```python
from build123d import *

# Parameters (mm, degrees)
F0_R     = 5
F1_DEPTH = 5
F2_R     = 1
F3_DEPTH = 1


with BuildPart() as f1:
    # F0 (on Front) → F1 (new body)
    with BuildSketch(Plane.XZ):
        with BuildLine():
            ThreePointArc((9.943923, -1.057539), (9.985971, -0.529512), (10, 0))
            ThreePointArc((10, 0), (9.985971, 0.529512), (9.943923, 1.057539))
            ThreePointArc((9.943923, 1.057539), (9.510565, 3.09017), (8.666409, 4.989325))
            ThreePointArc((8.666409, 4.989325), (8.09017, 5.877853), (7.423197, 6.700458))
            ThreePointArc((7.423197, 6.700458), (5.877853, 8.09017), (4.07862, 9.130436))
            ThreePointArc((4.07862, 9.130436), (3.09017, 9.510565), (2.067062, 9.784031))
            ThreePointArc((2.067062, 9.784031), (0, 10), (-2.067062, 9.784031))
            ThreePointArc((-2.067062, 9.784031), (-3.09017, 9.510565), (-4.07862, 9.130436))
            ThreePointArc((-4.07862, 9.130436), (-5.877853, 8.09017), (-7.423197, 6.700458))
            ThreePointArc((-7.423197, 6.700458), (-8.09017, 5.877853), (-8.666409, 4.989325))
            ThreePointArc((-8.666409, 4.989325), (-9.510565, 3.09017), (-9.943923, 1.057539))
            ThreePointArc((-9.943923, 1.057539), (-10, 0), (-9.943923, -1.057539))
            ThreePointArc((-9.943923, -1.057539), (-9.510565, -3.09017), (-8.666409, -4.989325))
            ThreePointArc((-8.666409, -4.989325), (-8.09017, -5.877853), (-7.423197, -6.700458))
            ThreePointArc((-7.423197, -6.700458), (-5.877853, -8.09017), (-4.07862, -9.130436))
            ThreePointArc((-4.07862, -9.130436), (-3.09017, -9.510565), (-2.067062, -9.784031))
            ThreePointArc((-2.067062, -9.784031), (0, -10), (2.067062, -9.784031))
            ThreePointArc((2.067062, -9.784031), (3.09017, -9.510565), (4.07862, -9.130436))
            ThreePointArc((4.07862, -9.130436), (5.877853, -8.09017), (7.423197, -6.700458))
            ThreePointArc((7.423197, -6.700458), (8.09017, -5.877853), (8.666409, -4.989325))
            ThreePointArc((8.666409, -4.989325), (9.510565, -3.09017), (9.943923, -1.057539))
        make_face()
        Circle(F0_R, mode=Mode.SUBTRACT)
        with BuildLine():
            ThreePointArc((8.666409, 4.989325), (9.510565, 3.09017), (9.943923, 1.057539))
            Line((9.943923, 1.057539), (12.82726, 2.590636))
            Line((12.82726, 2.590636), (11.900209, 5.443806))
            Line((11.900209, 5.443806), (8.666409, 4.989325))
        make_face()
        with BuildLine():
            Line((12.82726, -2.590636), (9.943923, -1.057539))
            ThreePointArc((9.943923, -1.057539), (9.510565, -3.09017), (8.666409, -4.989325))
            Line((8.666409, -4.989325), (11.900209, -5.443806))
            Line((11.900209, -5.443806), (12.82726, -2.590636))
        make_face()
        with BuildLine():
            ThreePointArc((4.07862, 9.130436), (5.877853, 8.09017), (7.423197, 6.700458))
            Line((7.423197, 6.700458), (8.854734, 9.635543))
            Line((8.854734, 9.635543), (6.427683, 11.398899))
            Line((6.427683, 11.398899), (4.07862, 9.130436))
        make_face()
        with BuildLine():
            Line((8.854734, -9.635543), (7.423197, -6.700458))
            ThreePointArc((7.423197, -6.700458), (5.877853, -8.09017), (4.07862, -9.130436))
            Line((4.07862, -9.130436), (6.427683, -11.398899))
            Line((6.427683, -11.398899), (8.854734, -9.635543))
        make_face()
        with BuildLine():
            ThreePointArc((-2.067062, 9.784031), (0, 10), (2.067062, 9.784031))
            Line((2.067062, 9.784031), (1.5, 13))
            Line((1.5, 13), (-1.5, 13))
            Line((-1.5, 13), (-2.067062, 9.784031))
        make_face()
        with BuildLine():
            Line((1.5, -13), (2.067062, -9.784031))
            ThreePointArc((2.067062, -9.784031), (0, -10), (-2.067062, -9.784031))
            Line((-2.067062, -9.784031), (-1.5, -13))
            Line((-1.5, -13), (1.5, -13))
        make_face()
        with BuildLine():
            ThreePointArc((-7.423197, 6.700458), (-5.877853, 8.09017), (-4.07862, 9.130436))
            Line((-4.07862, 9.130436), (-6.427683, 11.398899))
            Line((-6.427683, 11.398899), (-8.854734, 9.635543))
            Line((-8.854734, 9.635543), (-7.423197, 6.700458))
        make_face()
        with BuildLine():
            Line((-6.427683, -11.398899), (-4.07862, -9.130436))
            ThreePointArc((-4.07862, -9.130436), (-5.877853, -8.09017), (-7.423197, -6.700458))
            Line((-7.423197, -6.700458), (-8.854734, -9.635543))
            Line((-8.854734, -9.635543), (-6.427683, -11.398899))
        make_face()
        with BuildLine():
            ThreePointArc((-9.943923, 1.057539), (-9.510565, 3.09017), (-8.666409, 4.989325))
            Line((-8.666409, 4.989325), (-11.900209, 5.443806))
            Line((-11.900209, 5.443806), (-12.82726, 2.590636))
            Line((-12.82726, 2.590636), (-9.943923, 1.057539))
        make_face()
        with BuildLine():
            Line((-11.900209, -5.443806), (-8.666409, -4.989325))
            ThreePointArc((-8.666409, -4.989325), (-9.510565, -3.09017), (-9.943923, -1.057539))
            Line((-9.943923, -1.057539), (-12.82726, -2.590636))
            Line((-12.82726, -2.590636), (-11.900209, -5.443806))
        make_face()
    extrude(amount=F1_DEPTH)

    # F2 (on face) → F3 (join)
    with BuildSketch(Plane.XZ.offset(5)):
        with Locations((0, 8)):
            Circle(F2_R)
    extrude(amount=F3_DEPTH)


solid = f1.part
```
The listing builds one solid part. Answer for the finished solid, in the listing's coordinates (mm). A direction names the side the tool comes from. Give positions to 0.01 mm unless a question says otherwise; leave off trailing zeros. Order: outer loops, then holes, each group sorted by start corner. A loop starts at its lowest first (then second) coordinate and runs counter-clockwise, first axis right, second up.
1) Find section C-C on x = 3.25. Write down the section's boundary in (y, z).
Reported:
outline: (-5, -9.46) - (0, -9.46) - (0, -3.8) - (-5, -3.8) - close; (-5, 3.8) - (0, 3.8) - (0, 9.46) - (-5, 9.46) - close
2) Consider line 1 along Z through (x, y) = (0, -3.15); line 2 along Y through (x, z) = (0, 9.5); line 3 along Z through (x, y) = (1.25, -0.8). Determine where each line is inside the solid, lowest interval first.
Reported:
line 1: z = -13 to -5, 5 to 13
line 2: y = -5 to 0
line 3: z = -13 to -4.84, 4.84 to 13
3) Determine the mould class of faces 1 (the face through (-5.27, -2.46, -10.28)), 2 (the face through (3.104, -2.465, 9.506)), 3 (the face through (8.15, -2.46, -8.19)) for opening direction Z: pulls with the +Z half, pulls with the -Z half, needs draft (parallel to the pull), parting line crosses it, or undercut.
Reported:
face 1: pulls with the -Z half
face 2: pulls with the +Z half
face 3: undercut
4) For faces 4 (the face through (8, -2, 6)), 5 (the face through (11.406, -2.465, -1.835)), 6 (the face through (-11.365, -2.465, -1.813)), 7 (the face through (-3.076, -2.465, 9.515)), determine the directions among +Z, -Z, +X, -X, +Y, -Y from which every point of the face is accessible in a straight line to the end or side of a thin tool.
Reported:
face 4: +Y, -Y
face 5: +X, +Y, -Y
face 6: -X, +Y, -Y
face 7: +Z, +Y, -Y
5) Given P1, Ø5, axis at x = -3.5, z = 9, coming from the -Y side; P2, Ø1, axis at x = -10, z = 0, coming from the +Y side; P3, Ø8, axis at x = 0, z = 0, coming from the -Y side; P4, Ø1, axis at y = -4.5, z = -0.5, coming from the +X side, each flat-ended and moving along its own axis, determine where each tip first touches the part or whether it passes through.
Reported:
P1: stops at y = -5
P2: stops at y = 0
P3: passes through
P4: stops at x = 10
6) Find section D-D on x = 6. Write down the section's boundary in (y, z).
Reported:
outline: (-5, -10.99) - (0, -10.99) - (0, 10.99) - (-5, 10.99) - close
7) Find section A-A on x = 0. Write down the section's boundary in (y, z), then the cut area to 3 significant figures.
Reported:
outline: (-6, 7) - (-5, 7) - (-5, 5) - (0, 5) - (0, 13) - (-5, 13) - (-5, 9) - (-6, 9) - close; (-5, -13) - (0, -13) - (0, -5) - (-5, -5) - close
area: 82.0 mm2
8) Find section B-B on z = 8. Write down the section's boundary in (x, y).
Reported:
outline: (-8.06, -5) - (-1, -5) - (-1, -6) - (1, -6) - (1, -5) - (8.06, -5) - (8.06, 0) - (-8.06, 0) - close
